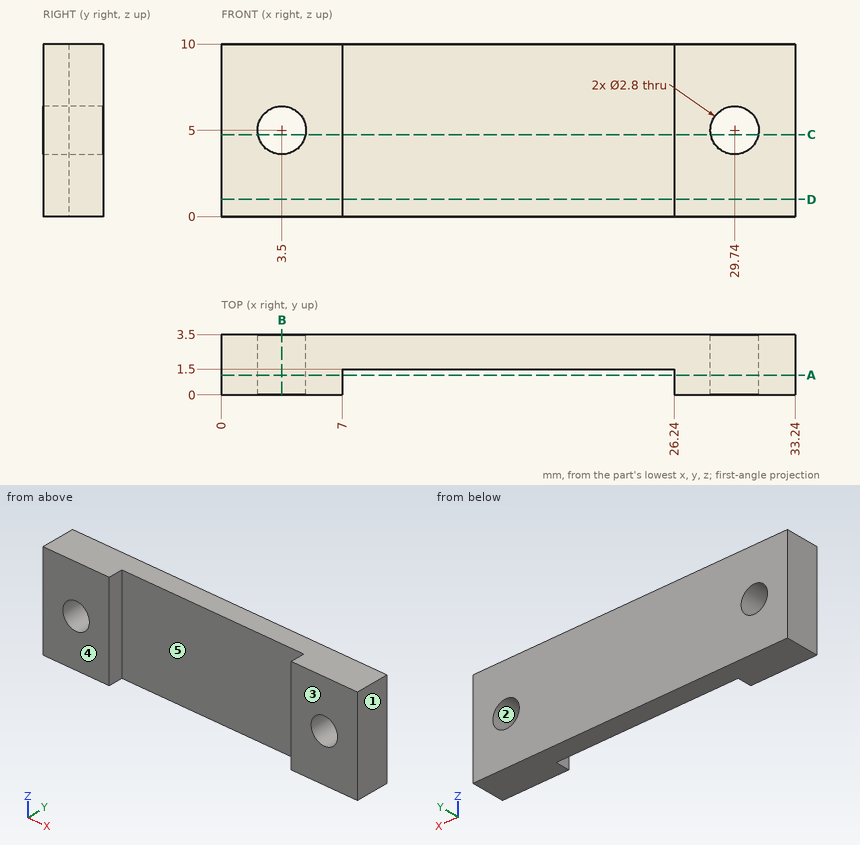
Geometry: see drawing. Coordinates: mm, zero at the bounding-box minimum. A direction names the side the tool comes from. Coordinates: 2 decimals unless noted, no trailing zeros. Loops run counter-clockwise (first coordinate to the right, second up) from the corner with the lowest first, then second, coordinate; pieces in that order, holes last.
(1) Pull-direction query (X, two-part tool) for the marked faces 1, 2 and 3; classes: released by +X, released by -X, zero draft, split by the parting line, or undercut.
(2) Section B-B on x = 3.5. Return the cut outline in (y, z), then the cut area to 3 significant figures.
(3) Section D-D on z = 1. Return the cut outline in (x, y).
(4) Material intervals for probe 1 along X at (y, z) = (2.25, 5); probe 2 along X at (y, z) = (1.15, 5); probe 3 along X at (y, z) = (1.65, 6), sorted ascending.
(5) First-contact query: pin 1 Ø1 at (x, z) = (6.5, 8.5) entering from -Y; pin 2 Ø4 at (x, z) = (18, 5.5) entering from -Y; pin 3 Ø2 at (x, z) = (29.74, 5) entering from -Y. Flat tips, straight axial feed; report the tip coordinate or a pass-through.
(6) Section C-C on z = 4.75. Return the cut outline in (x, y), then the cut area to 3 significant figures.
(7) Section A-A on y = 1.15. Return the cut outline in (x, z).
(8) Set-up query: the marked faces 4 and 5. Return all of +Z, -Z, +X, -X, +Y, -Y with unobstructed straight access to the full face (end or side cutting, diameter ignored); none if empty.
Data:
1. face 1: released by +X
1. face 2: undercut
1. face 3: zero draft
2. outline: (0, 0) - (3.5, 0) - (3.5, 3.6) - (0, 3.6) - close; (0, 6.4) - (3.5, 6.4) - (3.5, 10) - (0, 10) - close
2. area: 25.2 mm2
3. outline: (0, 0) - (7, 0) - (7, 1.5) - (26.24, 1.5) - (26.24, 0) - (33.24, 0) - (33.24, 3.5) - (0, 3.5) - close
4. probe 1: x = 0 to 2.1, 4.9 to 28.34, 31.14 to 33.24
4. probe 2: x = 0 to 2.1, 4.9 to 7, 26.24 to 28.34, 31.14 to 33.24
4. probe 3: x = 0 to 2.52, 4.48 to 28.76, 30.72 to 33.24
5. pin 1: stops at y = 0
5. pin 2: stops at y = 1.5
5. pin 3: passes through
6. outline: (0, 0) - (2.12, 0) - (2.12, 3.5) - (0, 3.5) - close; (4.88, 0) - (7, 0) - (7, 1.5) - (26.24, 1.5) - (26.24, 0) - (28.36, 0) - (28.36, 3.5) - (4.88, 3.5) - close; (31.12, 0) - (33.24, 0) - (33.24, 3.5) - (31.12, 3.5) - close
6. area: 68.2 mm2
7. outline: (0, 0) - (7, 0) - (7, 10) - (0, 10) - close; (26.24, 0) - (33.24, 0) - (33.24, 10) - (26.24, 10) - close; hole circle Ø2.8 at (3.5, 5); hole circle Ø2.8 at (29.74, 5)
8. face 4: +Z, -Z, +X, -X, -Y
8. face 5: +Z, -Z, -Y
